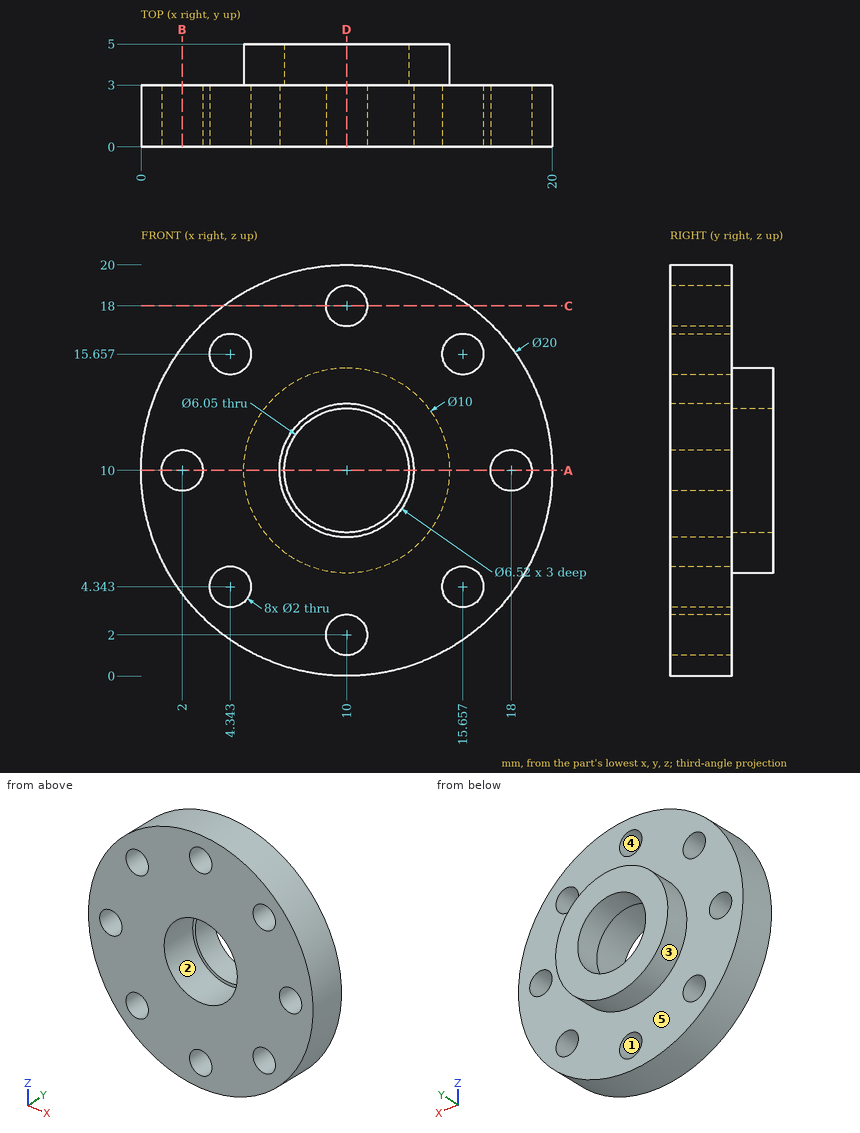
Print and shaded views of the part. All mm, measured from the part's lowest x, y and z. A direction names the side the tool comes from. Coordinates: 2 decimals unless noted, no trailing zeros. Loops run counter-clockwise (first coordinate to the right, second up) from the corner with the lowest first, then second, coordinate; pieces in that order, holes last. Notation, with made-up numbers: M -3,8 L 30,8 A20 ccw 30,24 Z; hole C -37.75,57 d6. An arc over 180 degrees is marked long. Use a Markdown table: item, result. Add a question column.
Q1. Cut at A-A (z = 10). Write the cut outline in (x, y) (3 decimals).
Q2. Cut at B-B (x = 2). Write the cut outline in (y, z).
Q3. Pin check, flat tips, straight feed: P1, Ø1.5, axis at x = 6.5, z = 4, coming from the +Y side; P2, Ø1.5, axis at y = 4.5, z = 14, coming from the -X side. Stop position of each tip, or through.
Q4. Probe L1, parallel to X at y = 1.2, z = 10; L2, parallel to Z at x = 10.75, y = 0.35; L3, parallel to X at y = 2.85, z = 5. List the from-to ranges inside material, lowest first.
Q5. Cut at D-D (x = 10). Write the cut outline in (y, z) (3 decimals).
Q6. Cut at C-C (z = 18). Write the cut outline in (x, y).
Q7. Which spindle directions (+Z, -Z, +X, -X, +Y, -Y) get a long thin tool onto all of the face, cutting with end or side? Do the marked faces 1 and 2. Say none if no direction does.
Q8. Mould opens along Z. For the marked faces 3, 4 and 5 say: +Z half, -Z half, draft (parallel to the pull), parting line (faces both ways), or undercut.
Worked out:
| question | item | result |
|---|---|---|
| 1 | outline | M 0,0 L 1,0 L 1,3 L 0,3 Z; M 3,0 L 6.74,0 L 6.74,3 L 6.975,3 L 6.975,5 L 5,5 L 5,3 L 3,3 Z; M 13.025,3 L 13.26,3 L 13.26,0 L 17,0 L 17,3 L 15,3 L 15,5 L 13.025,5 Z; M 19,0 L 20,0 L 20,3 L 19,3 Z |
| 2 | outline | M 0,4 L 3,4 L 3,9 L 0,9 Z; M 0,11 L 3,11 L 3,16 L 0,16 Z |
| 3 | P1 | stops at y = 3 |
| 3 | P2 | stops at x = 6.2 |
| 4 | L1 | x = 0 to 1, 3 to 6.74, 13.26 to 17, 19 to 20 |
| 4 | L2 | z = 0.03 to 1.34, 2.66 to 6.83, 13.17 to 17.34, 18.66 to 19.97 |
| 4 | L3 | x = 1.34 to 3.59, 5.1 to 14.9, 16.41 to 18.66 |
| 5 | outline | M 0,0 L 3,0 L 3,1 L 0,1 Z; M 0,3 L 3,3 L 3,5 L 5,5 L 5,6.975 L 3,6.975 L 3,6.74 L 0,6.74 Z; M 0,13.26 L 3,13.26 L 3,13.025 L 5,13.025 L 5,15 L 3,15 L 3,17 L 0,17 Z; M 0,19 L 3,19 L 3,20 L 0,20 Z |
| 6 | outline | M 4,0 L 9,0 L 9,3 L 4,3 Z; M 11,0 L 16,0 L 16,3 L 11,3 Z |
| 7 | face 1 | +Y, -Y |
| 7 | face 2 | -Y |
| 8 | face 3 | parting line |
| 8 | face 4 | undercut |
| 8 | face 5 | draft |
